Design review of the part built by this model. Coordinates are the model's own, in mm. Face numbers are marked on the shaded views. A direction names the side the tool comes from. Give positions to 0.01 mm unless a question says otherwise; leave off trailing zeros. Loops run counter-clockwise (first coordinate to the right, second up) from the corner with the lowest first, then second, coordinate; pieces in that order, holes last. Notation, with made-up numbers: (29.5, 78.5) -> (48.5, 78.5) arc R30 cw to (48.5, 117.5) -> close; hole circle Ø6 at (67.25, -23). An arc over 180 degrees is marked (long way). Answer in a Markdown table with one row per item. Add a question column.
(1) Consider section B-B on z = 20. Write out the cut boundary in (x, y), then the cut area to 3 significant figures.
(2) Draft analysis for pull direction Z (two halves, no side actions). For the marked faces 4, 5, 6 and 7, state which applies: +Z half, -Z half, draft (parallel to the pull), parting line (faces both ways), or undercut.
(3) Consider section A-A on x = 6. Write out the cut boundary in (y, z), then the cut area to 3 significant figures.
(4) For line 1 (X direction, y = -13.95, z = 20); line 2 (Z direction, x = 6, y = -14.45); line 3 (Z direction, x = 6, y = -13.5), list the stretches that pass through material, from the lowest coordinate up.
(5) Consider section D-D on y = 5.5. Write out the cut boundary in (x, z).
(6) Consider section C-C on x = 1.25. Write out the cut boundary in (y, z), then the cut area to 3 significant figures.
(7) For the marked faces 1, 2 and 3, list the 3-axis set-ups (+Z, -Z, +X, -X, +Y, -Y) from which the entire face can be reached by the end or side of a thin tool; tool diameter is ignored.
(8) For pin 1 (1 mm diameter, centred on x = 3.5, z = -8.5, fed in from +Y); pin 2 (5 mm diameter, centred on x = 9, y = 5.5, fed in from +Z); pin 3 (3 mm diameter, centred on x = 3, y = -11, fed in from +Z); pin 4 (3 mm diameter, centred on x = 6, z = 20, fed in from +Y), all flat-tipped, find the tip position at first contact; note any pin that passes through.
Autodesk Inventor part; units mm, degrees
ref_plane "YZ Plane" through (0, 0, 0) normal (1, 0, 0) x (0, 1, 0)
ref_plane "XZ Plane" through (0, 0, 0) normal (0, 1, 0) x (-1, 0, 0)
ref_plane "XY Plane" through (0, 0, 0) normal (0, 0, 1) x (1, 0, 0)
sketch "Sketch1" plane through (0, 0, 0) normal (1, 0, 0) x (0, 1, 0)
  circle A0 centre (0, 0) radius 7
  line L0 (0, 10) -> (-10.5, 10)
  line L1 (0, -10) -> (-10.5, -10)
  line L2 (-7.8658, 6.1749) -> (-12.5, 6.1749)
  line L3 (-15, 8.6749) -> (-15, 15.4804)
  arc A1 (-13, 12.5) -> (-10.5, 10) centre (-10.5, 12.5) ccw
  arc A2 (-15, 8.6749) -> (-12.5, 6.1749) centre (-12.5, 8.6749) ccw
  line L4 (-15, 20.163) -> (-15, 15.4804)
  line L5 (0, 0) -> (-13.6801, 0) construction
  line L6 (-7.8658, -6.1749) -> (-12.5, -6.1749)
  arc A3 (-7.8658, 6.1749) -> (-7.8658, -6.1749) centre (0, 0) ccw
  arc A4 (0, -10) -> (0, 10) centre (0, 0) ccw
  line L7 (-13, 12.5) -> (-13, 27.5)
  line L8 (-13, 27.5) -> (-15, 27.5)
  line L9 (-15, 27.5) -> (-15, 20.163)
  line L10 (-7.8658, -6.1749) -> (-12.5, -6.1749)
  line L11 (-15, -8.6749) -> (-15, -15.4804)
  arc A5 (-10.5, -10) -> (-13, -12.5) centre (-10.5, -12.5) ccw
  arc A6 (-12.5, -6.1749) -> (-15, -8.6749) centre (-12.5, -8.6749) ccw
  line L12 (-15, -20.163) -> (-15, -15.4804)
  line L13 (-13, -12.5) -> (-13, -27.5)
  line L14 (-15, -27.5) -> (-15, -20.163)
  line L15 (-13, -27.5) -> (-15, -27.5)
  point P0 (-13, 10)
  point P1 (-5.25, -10)
  point P2 (-13, -10)
  dimension "d0" = 14
  dimension "d2" = 13
  dimension "d4" = 2.5
  dimension "d7" = 15
extrude "Extrusion1" add sketch "Sketch1" along normal blind 12
sketch "Sketch2" plane through (0, -13, 27.5) normal (0, 1, 0) x (1, 0, 0)
  line L0 (0, 15) -> (0, 0) construction
  line L1 (0, 15) -> (12, 15) construction
  line L2 (0, 0) -> (12, 15) construction
  line L3 (12, 15) -> (12, 0) construction
  line L4 (0, 15) -> (12, 0) construction
  circle A0 centre (6, 7.5) radius 1.6
  point P0 (0, 27.5)
  dimension "d8" = 3.2
extrude "Extrusion2" cut sketch "Sketch2" against normal blind 12
sketch "Sketch3" plane through (0, -13, -12.5) normal (0, 1, 0) x (1, 0, 0)
  line L0 (12, -3.8251) -> (12, 15) construction
  line L1 (12, 15) -> (0, 0.0025) construction
  line L2 (0, -3.8251) -> (0, 15) construction
  line L3 (12, 0.0025) -> (0, 15) construction
  circle A0 centre (6, 7.5012) radius 1.6
  point P0 (0, -12.5)
  dimension "d11" = 3.2
extrude "Extrusion3" cut sketch "Sketch3" against normal blind 12
properties part number "Soporte_cojinete"
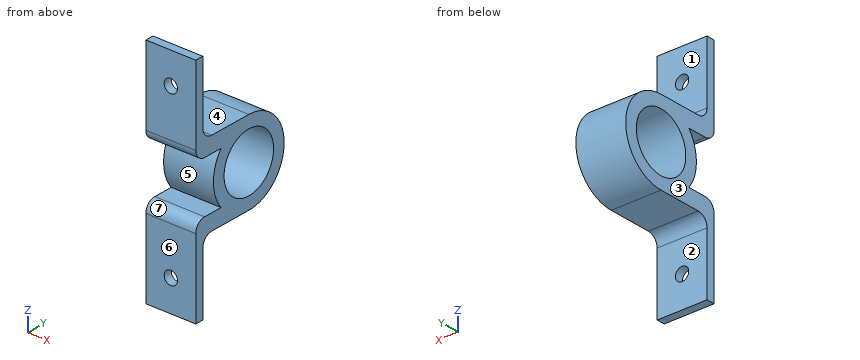
Values follow:
| question | item | result |
|---|---|---|
| 1 | outline | (0, -15) -> (4.4, -15) -> (4.4, -13) -> (0, -13) -> close; (7.6, -15) -> (12, -15) -> (12, -13) -> (7.6, -13) -> close |
| 1 | area | 17.6 mm2 |
| 2 | face 4 | +Z half |
| 2 | face 5 | undercut |
| 2 | face 6 | draft |
| 2 | face 7 | undercut |
| 3 | outline | (-15, -27.5) -> (-13, -27.5) -> (-13, -21.6) -> (-15, -21.6) -> close; (-15, -18.4) -> (-13, -18.4) -> (-13, -12.5) arc R2.5 cw to (-10.5, -10) -> (0, -10) arc R10 ccw to (0, 10) -> (-10.5, 10) arc R2.5 cw to (-13, 12.5) -> (-13, 18.4) -> (-15, 18.4) -> (-15, 8.67) arc R2.5 ccw to (-12.5, 6.17) -> (-7.87, 6.17) arc R10 ccw to (-7.87, -6.17) -> (-12.5, -6.17) arc R2.5 ccw to (-15, -8.67) -> close; (-15, 21.6) -> (-13, 21.6) -> (-13, 27.5) -> (-15, 27.5) -> close; hole circle Ø14 at (0, 0) |
| 3 | area | 290 mm2 |
| 4 | line 1 | 0 to 4.4, 7.6 to 12 |
| 4 | line 2 | -27.5 to -21.6, -18.4 to -7.11, 7.11 to 18.4, 21.6 to 27.5 |
| 4 | line 3 | -27.5 to -21.6, -18.4 to -6.38, 6.38 to 18.4, 21.6 to 27.5 |
| 5 | outline | (0, -8.35) -> (12, -8.35) -> (12, -4.33) -> (0, -4.33) -> close; (0, 4.33) -> (12, 4.33) -> (12, 8.35) -> (0, 8.35) -> close |
| 6 | outline | (-15, -27.5) -> (-13, -27.5) -> (-13, -12.5) arc R2.5 cw to (-10.5, -10) -> (0, -10) arc R10 ccw to (0, 10) -> (-10.5, 10) arc R2.5 cw to (-13, 12.5) -> (-13, 27.5) -> (-15, 27.5) -> (-15, 8.67) arc R2.5 ccw to (-12.5, 6.17) -> (-7.87, 6.17) arc R10 ccw to (-7.87, -6.17) -> (-12.5, -6.17) arc R2.5 ccw to (-15, -8.67) -> close; hole circle Ø14 at (0, 0) |
| 6 | area | 303 mm2 |
| 7 | face 1 | +Z, +X, -X, +Y |
| 7 | face 2 | -Z, +X, -X, +Y |
| 7 | face 3 | +Z, -Z, -X, +Y, -Y |
| 8 | pin 1 | y = 6 |
| 8 | pin 2 | z = 9.54 |
| 8 | pin 3 | z = 11 |
| 8 | pin 4 | through |
